from build123d import *

# Parameters (mm, degrees)
SKETCH001_W            = 5.018169
SKETCH001_H            = 3
EXTRUDE001_DEPTH       = 5
BOX_W                  = 210
BOX_H                  = 320
BOX_DEPTH              = 320
CUT001_PLACEMENT_ANGLE = 90
EXTRUDE_DEPTH          = 5


with BuildPart() as extrude001:
    # Sketch001 → Extrude001 (new body)
    with BuildSketch(Plane.XZ):
        with Locations((27.509085, -11.5)):
            Rectangle(SKETCH001_W, SKETCH001_H)
    extrude(amount=-EXTRUDE001_DEPTH)


with BuildPart() as cubo:
    # Box → Box (new body)
    with BuildSketch(Plane(origin=(0, -151, -150), x_dir=(1, 0, 0), z_dir=(0, 0, 1))):
        with Locations((105, 160)):
            Rectangle(BOX_W, BOX_H)
    extrude(amount=BOX_DEPTH)


with BuildPart() as cut:
    # Sphere → Sphere (revolve)
    with BuildSketch(Plane.XZ):
        with BuildLine():
            ThreePointArc((0, -150), (150, 0), (0, 150))
            Line((0, 150), (0, -150))
        make_face()
    revolve(axis=Axis((0, 0, 0), (0, 0, 1)))

    # Cut: cut Cubo
    add(cubo.part, mode=Mode.SUBTRACT)


with BuildPart() as cut001:
    # Sphere001 → Sphere001 (revolve)
    with BuildSketch(Plane.XZ):
        with BuildLine():
            ThreePointArc((0, -25), (25, 0), (0, 25))
            Line((0, 25), (0, -25))
        make_face()
    revolve(axis=Axis((0, 0, 0), (0, 0, 1)))

    # Cut001: cut Cut
    add(cut.part, mode=Mode.SUBTRACT)


with BuildPart() as cut001_1:
    # Cut001 placement: moved
    add(cut001.part.moved(Location((10, 0, -13))).rotate(Axis((10, 0, -13), (0, 1, 0)), CUT001_PLACEMENT_ANGLE))


with BuildPart() as fusion001:
    # Sketch → Extrude (new body)
    with BuildSketch(Plane.XZ):
        Polygon((0, 0), (25, 0), (25, -3), (30, -3), (30, 5), (-5, 5), (-5, -13), (0, -13), align=None)
    extrude(amount=-EXTRUDE_DEPTH)

    # Fusion: union Cut001
    add(cut001_1.part)

    # Fusion001: union Extrude001
    add(extrude001.part)


solid = fusion001.part
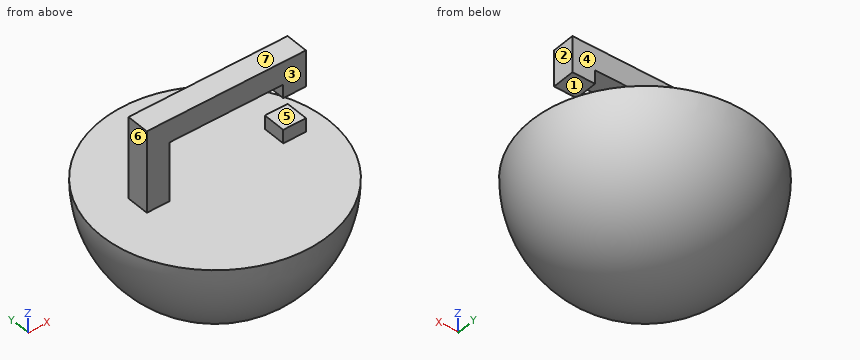
Check sheet for the modelled part. Datum: model origin and axes. Units: mm. Face numbers are marked on the shaded views. A direction names the side the tool comes from. Round coordinates to 2 decimals unless told otherwise and drop trailing zeros. Write each loop counter-clockwise with the first axis right and the second up, starting at its lowest first coordinate (ties: lowest second). Pieces come first, ordered by that corner, then holes. Notation, with made-up numbers: (67.5, 69.25) -> (112.5, 69.25) arc R13 cw to (112.5, 75.25) -> close; hole circle Ø7 at (55, -30). An arc over 180 degrees is marked (long way). Answer as CSV lines item,"result". Start each with the question number.
1) Section check A-A on z = -2. Enter the section's corners in (x, y), and give its area (3 significant figures).
2) Release check for a two-part mould opening along Z. For the marked faces 5, 6 and 7 record: pulls with the +Z half, pulls with the -Z half, needs draft (parallel to the pull), parting line crosses it, or undercut.
3) Section check B-B on x = 28. Enter the section's corners in (y, z), and give its area (3 significant figures).
4) Section check C-C on z = 2.5. Enter the section's corners in (x, y), and give its area (3 significant figures).
5) Go/stop test with flat-tipped pins: P1, Ø14.5, axis at x = 21, z = -5.5, coming from the -Y side; P2, Ø14.5, axis at x = 14, z = -3.5, coming from the +Y side; P3, Ø3.5, axis at y = 2.5, z = -11.5, coming from the -X side; P4, Ø10, axis at x = 13.5, z = -7, coming from the +Y side. Record where each tip stops, or that it passes through.
6) Material ranges on line 1 (Y direction, x = 23, z = 2); line 2 (X direction, y = 1, z = -4.5); line 3 (Y direction, x = -3.5, z = -25), recorded low to high. Write a range as from..to.
7) Section check D-D on y = 21. Enter the section's corners in (x, z).
8) Tool access check on the marked faces 1, 2, 3 and 4. Record the directions out of +Z, -Z, +X, -X, +Y, -Y that give a thin tool (end or side, any length) a straight path to the whole face; none if there is none.
Found:
1,outline,"(-5, 0) -> (0, 0) -> (0, 5) -> (-5, 5) -> close; (25, 0) -> (30, 0) -> (30, 5) -> (25, 5) -> close"
1,area,"50.0 mm^2"
2,face 5,"undercut"
2,face 6,"needs draft"
2,face 7,"pulls with the +Z half"
3,outline,"(-17.35, -13) arc R17.35 ccw to (17.35, -13) -> (5, -13) -> (5, -10) -> (0, -10) -> (0, -13) -> close; (0, -3) -> (5, -3) -> (5, 5) -> (0, 5) -> close"
3,area,"528 mm^2"
4,outline,"(-5, 0) -> (30, 0) -> (30, 5) -> (-5, 5) -> close"
4,area,"175 mm^2"
5,P1,"stops at y = 0"
5,P2,"stops at y = 5"
5,P3,"stops at x = -14.95"
5,P4,"passes through"
6,line 1,"y = 0..5"
6,line 2,"x = -5..0"
6,line 3,"y = -17.28..17.28"
7,outline,"(-3.56, -13) arc R13.56 ccw to (23.56, -13) -> close"
8,face 1,"+X, +Y, -Y"
8,face 2,"+Z, +X, +Y, -Y"
8,face 3,"+Z, +X, -X, -Y"
8,face 4,"+Z, +X, -X, +Y"
